Work out the finished part from the listing and answer in its coordinate system (mm). A direction names the side the tool comes from. Coordinates: 2 decimals unless noted, no trailing zeros. Order: outer loops, then holes, each group sorted by start corner. A loop starts at its lowest first (then second) coordinate and runs counter-clockwise, first axis right, second up. Notation, with made-up numbers: M -38.5,12.25 L -12.5,12.25 A14 cw -12.5,24.25 Z; hole C 43,29.25 d6. An arc over 180 degrees is marked long. Use a Markdown table: item, result.
from build123d import *

# Parameters (mm, degrees)
SKETCH_R        = 15
PAD_DEPTH       = 80
POCKET_DEPTH    = 63.001
FILLET_R        = 10
POCKET001_DEPTH = 45
FILLET001_R     = 4
SKETCH003_R     = 15
PAD001_DEPTH    = 40


with BuildPart() as part:
    # Sketch → Pad (new body)
    with BuildSketch(Plane.XY):
        with BuildLine():
            ThreePointArc((-18, 24), (0, -30), (18, 24))
            Line((18, 24), (18, 147))
            Line((18, 147), (-18, 147))
            Line((-18, 147), (-18, 24))
        make_face()
        Circle(SKETCH_R, mode=Mode.SUBTRACT)
    extrude(amount=PAD_DEPTH)

    # Sketch001 (on Face2 of Pad) → Pocket (cut, through all)
    with BuildSketch(Plane(origin=(33, 0, 40), x_dir=(0, 1, 0), z_dir=(1, 0, 0))):
        with BuildLine():
            Line((-34, -18), (36, -18))
            ThreePointArc((36, -18), (54, 0), (36, 18))
            Line((36, 18), (-34, 18))
            Line((-34, 18), (-34, -18))
        make_face()
        with BuildLine():
            ThreePointArc((36, -40), (56.976177, -34.058773), (71.721142, -18))
            Line((147, -18), (71.721142, -18))
            Line((147, -18), (147, -40))
            Line((147, -40), (36, -40))
        make_face()
        with BuildLine():
            Line((147, 18), (71.721142, 18))
            ThreePointArc((71.721142, 18), (56.976177, 34.058773), (36, 40))
            Line((147, 40), (36, 40))
            Line((147, 18), (147, 40))
        make_face()
    extrude(amount=-POCKET_DEPTH, mode=Mode.SUBTRACT)

    # Fillet
    fillet_edges = [part.edges().sort_by_distance(p)[0] for p in [
        (0, 71.721142, 58),
        (0, 71.721142, 22),
    ]]
    fillet(fillet_edges, radius=FILLET_R)

    # Sketch002 (on Face7 of Fillet) → Pocket001 (cut)
    with BuildSketch(Plane(origin=(0, 147, 0), x_dir=(-1, 0, 0), z_dir=(0, 1, 0))):
        Polygon((-18, 58), (-10.928932, 58), (-18, 50.928932), align=None)
        Polygon((-18, 22), (-10.928932, 22), (-18, 29.071068), align=None)
        Polygon((18, 22), (10.928932, 22), (18, 29.071068), align=None)
        Polygon((18, 58), (10.928932, 58), (18, 50.928932), align=None)
    extrude(amount=-POCKET001_DEPTH, mode=Mode.SUBTRACT)

    # Fillet001
    fillet001_edges = [part.edges().sort_by_distance(p)[0] for p in [
        (-14.464466, 102, 25.535534),
        (14.464466, 102, 25.535534),
        (-14.464466, 102, 54.464466),
        (14.464466, 102, 54.464466),
    ]]
    fillet(fillet001_edges, radius=FILLET001_R)

    # Sketch003 (on Face7 of Fillet001) → Pad001 (join)
    with BuildSketch(Plane(origin=(0, 147, 40), x_dir=(-1, 0, 0), z_dir=(0, 1, 0))):
        Circle(SKETCH003_R)
    extrude(amount=PAD001_DEPTH)


solid = part.part
(1) A cutting plane is placed at A-A (y = 0). Determine the outline of the cut face in (x, z), then the cut area to 3 significant figures.
Conclusion:
| item | result |
|---|---|
| outline | M -30,0 L -15,0 L -15,22 L -30,22 Z; M -30,58 L -15,58 L -15,80 L -30,80 Z; M 15,0 L 30,0 L 30,22 L 15,22 Z; M 15,58 L 30,58 L 30,80 L 15,80 Z |
| area | 1,320 mm2 |
(2) Straight lines are drawn through the part: L1, parallel to X at y = 0, z = 68; L2, parallel to Z at x = 23, y = 18.5; L3, parallel to Z at x = -9.5, y = 133.5. For each, find the intervals that lie inside material, in ascending order.
Conclusion:
| item | result |
|---|---|
| L1 | -30 to -15, 15 to 30 |
| L2 | 0 to 22, 58 to 80 |
| L3 | 22 to 58 |
(3) A cutting plane is placed at B-B (x = 0). Determine the outline of the cut face in (y, z).
Conclusion:
| item | result |
|---|---|
| outline | M -30,0 L -15,0 L -15,22 L -30,22 Z; M -30,58 L -15,58 L -15,80 L -30,80 Z; M 15,0 L 36,0 A40 ccw 69.14,17.6 A10 cw 77.42,22 L 147,22 L 147,25 L 187,25 L 187,55 L 147,55 L 147,58 L 77.42,58 A10 cw 69.14,62.4 A40 ccw 36,80 L 15,80 L 15,58 L 36,58 A18 cw 36,22 L 15,22 Z |
(4) Which of the six approach directions +Z, -Z, +X, -X, +Y, -Y give full straight-line access (tool end or side, diameter ignored) to faces 4 (the flat face through (14.415, 126.787, 54.514)), 5 (the flat face through (-14.415, 126.787, 25.486)), 6 (the flat face through (0, 147, 56))?
Conclusion:
| item | result |
|---|---|
| face 4 | +Z, +X, +Y |
| face 5 | -Z, -X, +Y |
| face 6 | +Y |
(5) A cutting plane is placed at C-C (z = 40). Determine the outline of the cut face in (x, y).
Conclusion:
| item | result |
|---|---|
| outline | M -18,54 L 18,54 L 18,147 L 15,147 L 15,187 L -15,187 L -15,147 L -18,147 Z |
(6) A cutting plane is placed at D-D (x = 23.5). Determine the outline of the cut face in (y, z), then the cut area to 3 significant figures.
Conclusion:
| item | result |
|---|---|
| outline | M -18.65,0 L 18.65,0 L 18.65,22 L -18.65,22 Z; M -18.65,58 L 18.65,58 L 18.65,80 L -18.65,80 Z |
| area | 1,640 mm2 |
(7) Given P1, Ø6, axis at x = -15.5, y = 137.5, coming from the +Z side; P2, Ø3, axis at y = 127.5, z = 36.5, coming from the +X side; P3, Ø3, axis at x = -6, z = 66, coming from the -Y side, each flat-ended and moving along its own axis, determine where each tip first touches the part or whether it passes through.
Conclusion:
| item | result |
|---|---|
| P1 | z = 56.43 |
| P2 | x = 18 |
| P3 | y = -29.66 |
(8) Determine the mould class of faces 1 (the cylindrical face through (1.953, 166.72, 54.872)), 2 (the flat face through (0, 18, 58)), 3 (the cylindrical face through (-0.25, 72.79, 59.14)) for opening direction Z: pulls with the +Z half, pulls with the -Z half, needs draft (parallel to the pull), parting line crosses it, or undercut.
Conclusion:
| item | result |
|---|---|
| face 1 | parting line crosses it |
| face 2 | undercut |
| face 3 | pulls with the +Z half |
